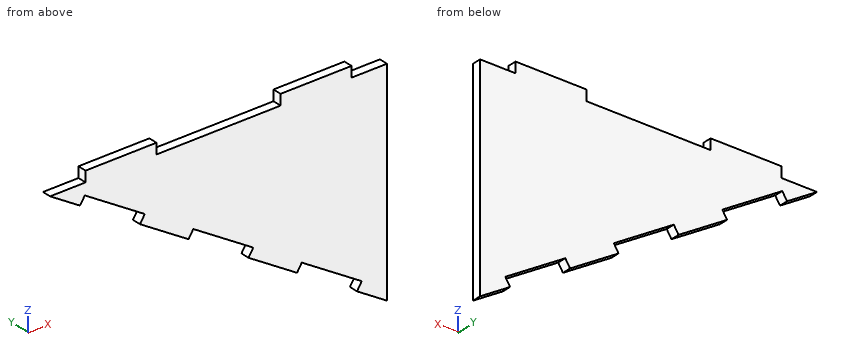
```python
from build123d import *

# Parameters (mm, degrees)
F0_W     = 25.4
F0_H     = 3.785962
F1_DEPTH = 3.175


with BuildPart() as f1:
    # F0 (on Front) → F1 (new body)
    with BuildSketch(Plane.XZ):
        with Locations((32.3196, 1.892981)):
            Rectangle(F0_W, F0_H)
        Polygon((-50.2304, 0), (-62.9304, 0), (-52.192691, -6.781711), (-50.497263, -4.097284), (-29.021845, -17.660706), (-30.717273, -20.345133), (-13.343109, -31.318289), (-11.647681, -28.633862), (-0.909972, -35.415573), (9.827737, -42.197284), (8.132309, -44.881711), (25.506473, -55.854867), (27.201901, -53.17044), (48.677319, -66.733862), (46.981891, -69.418289), (57.7196, -76.2), (57.7196, 0), (45.0196, 0), (19.6196, 0), (-24.8304, 0), align=None)
        with Locations((-37.5304, 1.892981)):
            Rectangle(F0_W, F0_H)
    extrude(amount=F1_DEPTH)


solid = f1.part
```
The listing builds one solid part. Answer for the finished solid, in the listing's coordinates (mm). Coordinates: 2 decimals unless noted, no trailing zeros. Loops run counter-clockwise (first coordinate to the right, second up) from the corner with the lowest first, then second, coordinate; pieces in that order, holes last. Notation, with made-up numbers: M -20.75,19.5 L -5.75,19.5 A34 cw -5.75,54.5 Z; hole C 59.25,5.5 d10. An arc over 180 degrees is marked long. Answer as CSV lines item,"result". Start each with the question number.
(1) The part is cut by section A-A (y = -2.1). Give the vertices of the cut face in (x, z), and give its area (3 significant figures).
(2) The part is cut by section B-B (x = -8.5). Give the vertices of the cut face in (y, z) (3 decimals), and give its area (3 significant figures).
(3) Find the intervals of material crossed by L1, parallel to Z at x = 47.5, y = -0.4; L2, parallel to Z at x = -56, y = -2.1; L3, parallel to Z at x = 2, y = -2.35, in increasing order. Write a range as [from, to].
(4) Given pin 1 (1 mm diameter, centred on x = -7, y = -1, fed in from +Z); pin 2 (1 mm diameter, centred on x = 1, y = -0.5, fed in from -Z); pin 3 (1.6 mm diameter, centred on y = -2.5, z = 1.5, fed in from +X), each flat-ended and moving along its own axis, determine where each tip first touches the part or whether it passes through.
(5) The part is cut by section C-C (z = -64). Give the vertices of the cut face in (x, y) (3 decimals).
Determined:
1,outline,"M -62.93,0 L -52.19,-6.78 L -50.5,-4.1 L -29.02,-17.66 L -30.72,-20.35 L -13.34,-31.32 L -11.65,-28.63 L 9.83,-42.2 L 8.13,-44.88 L 25.51,-55.85 L 27.2,-53.17 L 48.68,-66.73 L 46.98,-69.42 L 57.72,-76.2 L 57.72,0 L 45.02,0 L 45.02,3.79 L 19.62,3.79 L 19.62,0 L -24.83,0 L -24.83,3.79 L -50.23,3.79 L -50.23,0 Z"
1,area,"4,550 mm2"
2,outline,"M -3.175,-30.622 L 0,-30.622 L 0,0 L -3.175,0 Z"
2,area,"97.2 mm2"
3,L1,"[-69.75, -68.6], [-65.99, 0]"
3,L2,"[-4.38, 0]"
3,L3,"[-37.25, 0]"
4,pin 1,"z = 0"
4,pin 2,"z = -36.94"
4,pin 3,"x = 45.02"
5,outline,"M 44.349,-3.175 L 57.72,-3.175 L 57.72,0 L 44.349,0 Z"
